Could you check a few things on this model? Use its own coordinates, in mm. Give positions to 0.01 mm unless a question says otherwise; leave off trailing zeros. Loops run counter-clockwise (first coordinate to the right, second up) from the corner with the lowest first, then second, coordinate; pieces in that order, holes last. Notation, with made-up numbers: M -16.5,4 L 15.5,4 A26 cw 15.5,32 Z; hole C 10.5,-34 d10. An arc over 180 degrees is marked long. Answer in a Markdown table with one row per item. Add a question column.
1. If we section it at C-C on x = 70: List the corners of the cut face in (y, z) for me, then the cut area to 3 significant figures.
2. I need wall thicknesses on line 1 along X through (y, z) = (133, 1.65); line 2 along X through (y, z) = (9, 2.7); line 3 along Y through (x, z) = (-111, 2.4). Which ranges of each line are inside material? Lowest first, please. Write a range as from..to.
3. If we section it at D-D on y = 145.5: List the corners of the cut face in (x, z) for me, then the cut area to 3 significant figures.
4. If we section it at B-B on z = 3.9: Count the separate pieces of the cut face and the enclosed holes in it, then the cut area to 3 significant figures.
5. I'm going to push flat-ended pins straight in: pin 1 Ø2.5 at (y, z) = (17.5, 1.5) entering from +X; pin 2 Ø2.5 at (y, z) = (18.5, 2.5) entering from -X; pin 3 Ø3 at (x, y) = (23, 136.5) entering from +Z; pin 4 Ø1.5 at (x, z) = (184, 1.5) entering from +Y. Where does each tip first touch, or does it pass through?
6. If we section it at A-A on y = 110: List the corners of the cut face in (x, z) for me.
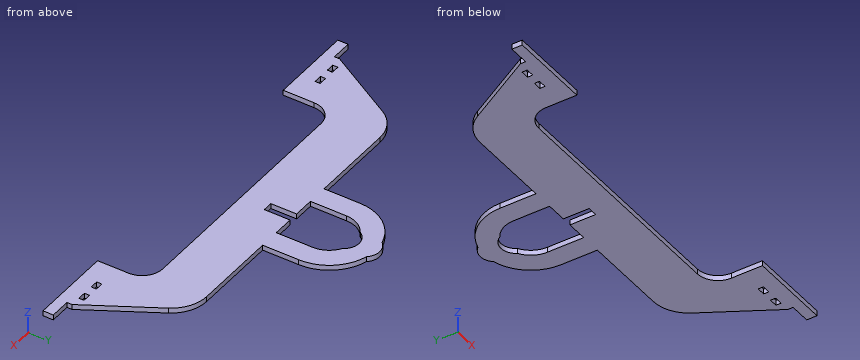
```python
from build123d import *

# Parameters (mm, degrees)
EXTRUDE_1_DEPTH     = 5
CUT_EXTRUDE_1_REACH = 7
EXTRUDE_2_DEPTH     = 5
CUT_EXTRUDE_2_REACH = 7
SKETCH_4_W          = 9.6
SKETCH_4_H          = 50
EXTRUDE_3_DEPTH     = 5
CUT_EXTRUDE_3_REACH = 7
SKETCH_6_W          = 8
SKETCH_6_H          = 5


with BuildPart() as part:
    # 草图1 → 凸台-拉伸1 (new body)
    with BuildSketch(Plane.XY):
        Polygon((-216, 0), (-216, 10), (-196, 10), (-196, 15), (-146.925227119, 100), (146.925227119, 100), (196, 15), (196, 10), (216, 10), (216, 0), (136, 0), (136, 50), (-136, 50), (-136, 0), align=None)
    extrude(amount=EXTRUDE_1_DEPTH)

    # 草图2 → 切除-拉伸1 (cut, up to next)
    with BuildSketch(Plane.XY.offset(5), mode=Mode.PRIVATE) as cut_extrude_1_sk1:
        with BuildLine():
            Line((-146.925227119, 100), (-126.925227119, 100))
            ThreePointArc((-126.925227119, 100), (-144.245735195, 95.358983849), (-156.925227119, 82.679491924))
            Line((-156.925227119, 82.679491924), (-146.925227119, 100))
        make_face()
    cut_extrude_1_tool1 = extrude(cut_extrude_1_sk1.sketch, amount=-CUT_EXTRUDE_1_REACH, mode=Mode.PRIVATE) & part.part
    add(cut_extrude_1_tool1.solids().sort_by_distance((-144.827064, 96.365874, 5))[0], mode=Mode.SUBTRACT)
    # 草图2 → 切除-拉伸1 (cut, up to next)
    with BuildSketch(Plane.XY.offset(5), mode=Mode.PRIVATE) as cut_extrude_1_sk2:
        with BuildLine():
            Line((146.925227119, 100), (156.925227119, 82.679491924))
            ThreePointArc((156.925227119, 82.679491924), (144.245735195, 95.358983849), (126.925227119, 100))
            Line((126.925227119, 100), (146.925227119, 100))
        make_face()
    cut_extrude_1_tool2 = extrude(cut_extrude_1_sk2.sketch, amount=-CUT_EXTRUDE_1_REACH, mode=Mode.PRIVATE) & part.part
    add(cut_extrude_1_tool2.solids().sort_by_distance((144.827064, 96.365874, 5))[0], mode=Mode.SUBTRACT)

    # 草图3 → 凸台-拉伸2 (add)
    with BuildSketch(Plane.XY.offset(5)):
        with BuildLine():
            Line((-116, 50), (-136, 50))
            Line((-136, 50), (-136, 30))
            ThreePointArc((-136, 30), (-130.142135624, 44.142135624), (-116, 50))
        make_face()
        with BuildLine():
            Line((136, 50), (136, 30))
            ThreePointArc((136, 30), (130.142135624, 44.142135624), (116, 50))
            Line((116, 50), (136, 50))
        make_face()
    extrude(amount=-EXTRUDE_2_DEPTH)

    # 草图4 → 切除-拉伸2 (cut, up to next)
    with BuildSketch(Plane.XY.offset(5), mode=Mode.PRIVATE) as cut_extrude_2_sk1:
        with Locations((0, 100)):
            Rectangle(SKETCH_4_W, SKETCH_4_H)
    cut_extrude_2_tool1 = extrude(cut_extrude_2_sk1.sketch, amount=-CUT_EXTRUDE_2_REACH, mode=Mode.PRIVATE) & part.part
    add(cut_extrude_2_tool1.solids().sort_by_distance((0, 100, 5))[0], mode=Mode.SUBTRACT)

    # 草图5 → 凸台-拉伸3 (add)
    with BuildSketch(Plane(origin=(0, 0, 0), x_dir=(-1, 0, 0), z_dir=(0, 0, -1))):
        with BuildLine():
            Line((45, 100), (45, 135))
            ThreePointArc((45, 135), (35.642806819, 162.469807463), (11.462652354, 178.515601811))
            ThreePointArc((11.462652354, 178.515601811), (0, 183.840499693), (-11.462652354, 178.515601811))
            ThreePointArc((-11.462652354, 178.515601811), (-35.642806819, 162.469807463), (-45, 135))
            Line((-45, 135), (-45, 100))
            Line((-45, 100), (-25, 100))
            Line((-25, 100), (-25, 135))
            ThreePointArc((-25, 135), (-21.786738765, 147.261240312), (-12.97295888, 156.370595169))
            ThreePointArc((-12.97295888, 156.370595169), (0, 163.840499693), (12.97295888, 156.370595169))
            ThreePointArc((12.97295888, 156.370595169), (21.786738765, 147.261240312), (25, 135))
            Line((25, 135), (25, 100))
            Line((25, 100), (45, 100))
        make_face()
    extrude(amount=-EXTRUDE_3_DEPTH)

    # 草图6 → 切除-拉伸3 (cut, up to next)
    with BuildSketch(Plane.XY.offset(5), mode=Mode.PRIVATE) as cut_extrude_3_sk1:
        with Locations((-182, 17.5)):
            Rectangle(SKETCH_6_W, SKETCH_6_H)
    cut_extrude_3_tool1 = extrude(cut_extrude_3_sk1.sketch, amount=-CUT_EXTRUDE_3_REACH, mode=Mode.PRIVATE) & part.part
    add(cut_extrude_3_tool1.solids().sort_by_distance((-182, 17.5, 5))[0], mode=Mode.SUBTRACT)
    # 草图6 → 切除-拉伸3 (cut, up to next)
    with BuildSketch(Plane.XY.offset(5), mode=Mode.PRIVATE) as cut_extrude_3_sk2:
        with Locations((-164, 17.5)):
            Rectangle(SKETCH_6_W, SKETCH_6_H)
    cut_extrude_3_tool2 = extrude(cut_extrude_3_sk2.sketch, amount=-CUT_EXTRUDE_3_REACH, mode=Mode.PRIVATE) & part.part
    add(cut_extrude_3_tool2.solids().sort_by_distance((-164, 17.5, 5))[0], mode=Mode.SUBTRACT)
    # 草图6 → 切除-拉伸3 (cut, up to next)
    with BuildSketch(Plane.XY.offset(5), mode=Mode.PRIVATE) as cut_extrude_3_sk3:
        with Locations((182, 17.5)):
            Rectangle(SKETCH_6_W, SKETCH_6_H)
    cut_extrude_3_tool3 = extrude(cut_extrude_3_sk3.sketch, amount=-CUT_EXTRUDE_3_REACH, mode=Mode.PRIVATE) & part.part
    add(cut_extrude_3_tool3.solids().sort_by_distance((182, 17.5, 5))[0], mode=Mode.SUBTRACT)
    # 草图6 → 切除-拉伸3 (cut, up to next)
    with BuildSketch(Plane.XY.offset(5), mode=Mode.PRIVATE) as cut_extrude_3_sk4:
        with Locations((164, 17.5)):
            Rectangle(SKETCH_6_W, SKETCH_6_H)
    cut_extrude_3_tool4 = extrude(cut_extrude_3_sk4.sketch, amount=-CUT_EXTRUDE_3_REACH, mode=Mode.PRIVATE) & part.part
    add(cut_extrude_3_tool4.solids().sort_by_distance((164, 17.5, 5))[0], mode=Mode.SUBTRACT)


solid = part.part
```
Results:
| question | item | result |
|---|---|---|
| 1 | outline | M 50,0 L 100,0 L 100,5 L 50,5 Z |
| 1 | area | 250 mm2 |
| 2 | line 1 | -45..-25, 25..45 |
| 2 | line 2 | -216..-136, 136..216 |
| 2 | line 3 | 50..100 |
| 3 | outline | M -43.76,0 L -22.69,0 L -22.69,5 L -43.76,5 Z; M 22.69,0 L 43.76,0 L 43.76,5 L 22.69,5 Z |
| 3 | area | 211 mm2 |
| 4 | separate pieces | 1 |
| 4 | enclosed holes | 5 |
| 4 | area | 25,100 mm2 |
| 5 | pin 1 | x = 195.28 |
| 5 | pin 2 | x = -194.7 |
| 5 | pin 3 | through |
| 5 | pin 4 | y = 37.08 |
| 6 | outline | M -45,0 L -25,0 L -25,5 L -45,5 Z; M 25,0 L 45,0 L 45,5 L 25,5 Z |
